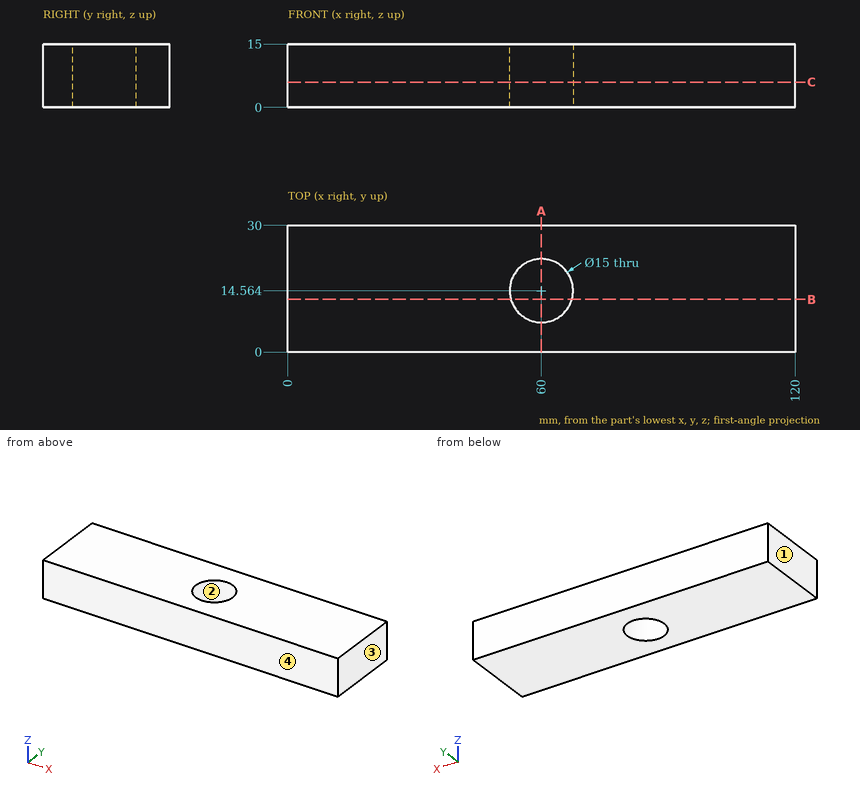
Answer from the drawing. Dimensions are ordinates in mm from the lowest x, y and z of the part. Give positions to 0.01 mm unless a question says otherwise; leave off trailing zeros. Order: outer loops, then holes, each group sorted by start corner. A loop starts at its lowest first (then second) coordinate and runs counter-clockwise, first axis right, second up. Notation, with made-up numbers: (-29, 50.5) -> (18, 50.5) arc R29 cw to (18, 84.5) -> close; hole circle Ø6 at (51, 4.25). An arc over 180 degrees is marked (long way). One line per item, written item: value. Start each with the question number.
(1) The part is cut by section A-A (x = 60). Determine the outline of the cut face in (y, z) (1 decimal), and give its area (3 significant figures).
(2) The part is cut by section C-C (z = 6). Determine the outline of the cut face in (x, y) (1 decimal), and give its area (3 significant figures).
(3) The part is cut by section B-B (y = 12.5). Determine the outline of the cut face in (x, z), and give its area (3 significant figures).
(4) Straight lines are drawn through the part: L1, parallel to X at y = 14.25, z = 2.75; L2, parallel to Y at x = 60, z = 3.5 (1 decimal); L3, parallel to X at y = 20.25, z = 1.5. For each, find the intervals that lie inside material, in ascending order.
(5) For a pull along X with two mould halves and no side action, classify the marked faces 1, 2, 3 and 4 as released by +X, released by -X, zero draft, split by the parting line, or undercut.
Taken from the geometry:
1. outline: (0, 0) -> (7.1, 0) -> (7.1, 15) -> (0, 15) -> close; (22.1, 0) -> (30, 0) -> (30, 15) -> (22.1, 15) -> close
1. area: 225 mm^2
2. outline: (0, 0) -> (120, 0) -> (120, 30) -> (0, 30) -> close; hole circle Ø15 at (60, 14.6)
2. area: 3,420 mm^2
3. outline: (0, 0) -> (52.79, 0) -> (52.79, 15) -> (0, 15) -> close; (67.21, 0) -> (120, 0) -> (120, 15) -> (67.21, 15) -> close
3. area: 1,580 mm^2
4. L1: 0 to 52.51, 67.49 to 120
4. L2: 0 to 7.1, 22.1 to 30
4. L3: 0 to 55.11, 64.89 to 120
5. face 1: released by -X
5. face 2: undercut
5. face 3: released by +X
5. face 4: zero draft
